from build123d import *

# Parameters (mm, degrees)
SKETCH1_R           = 24.15
SKETCH1_R_2         = 20.3
BOSS_EXTRUDE1_DEPTH = 70
CUT_EXTRUDE1_START  = -3.2
SKETCH2_R           = 21.65
SKETCH2_R_2         = 20.3
CUT_EXTRUDE1_DEPTH  = 3.2
SKETCH3_R           = 60
SKETCH3_R_2         = 8.4
BOSS_EXTRUDE2_DEPTH = 10


with BuildPart() as part:
    # Sketch1 → Boss-Extrude1 (new body)
    with BuildSketch(Plane.XY):
        Circle(SKETCH1_R)
        Circle(SKETCH1_R_2, mode=Mode.SUBTRACT)
    extrude(amount=BOSS_EXTRUDE1_DEPTH)

    # Sketch2 → Cut-Extrude1 (cut)
    with BuildSketch(Plane.XY.offset(70).offset(CUT_EXTRUDE1_START)):
        Circle(SKETCH2_R)
        Circle(SKETCH2_R_2, mode=Mode.SUBTRACT)
    extrude(amount=CUT_EXTRUDE1_DEPTH, mode=Mode.SUBTRACT)

    # Sketch3 → Boss-Extrude2 (add)
    with BuildSketch(Plane.XY.offset(70)):
        Circle(SKETCH3_R)
        Circle(SKETCH3_R_2, mode=Mode.SUBTRACT)
    extrude(amount=BOSS_EXTRUDE2_DEPTH)


solid = part.part
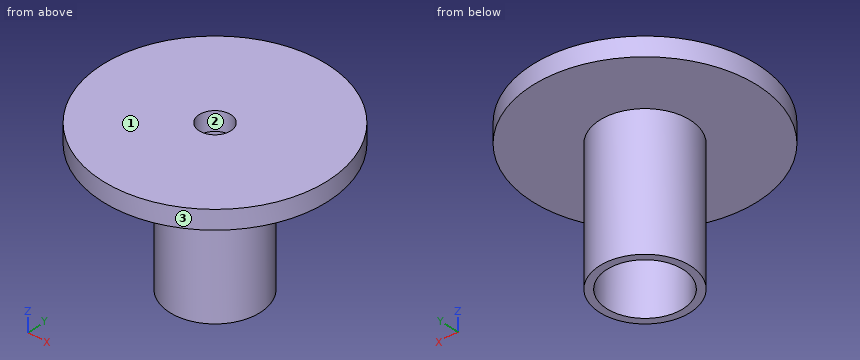
CAD build for the part. Positions are in the model's coordinates, mm. Face numbers are marked on the shaded views. Round coordinates to 2 decimals unless told otherwise and drop trailing zeros. Order: outer loops, then holes, each group sorted by start corner. A loop starts at its lowest first (then second) coordinate and runs counter-clockwise, first axis right, second up. Notation, with made-up numbers: (7, 53.5) -> (13, 53.5) arc R28 ccw to (13, 89.5) -> close; hole circle Ø8 at (-6, 67.25). An arc over 180 degrees is marked (long way). Write each question's results on one line, items separated by ' | '.
1. Cut at C-C (z = 74). Give the cut face in (x, y).
Findings below:
outline: circle Ø120 at (0, 0); hole circle Ø16.8 at (0, 0)
2. Wall check: line 1 along Y through (x, z) = (0, 74); line 2 along Y through (x, z) = (0, 67.7); line 3 along Z through (x, y) = (-8, 19). Give the ranges that are in metal, low to high. Write a range as [from, to].
Findings below:
line 1: y = [-60, -8.4], [8.4, 60] | line 2: y = [-24.15, -21.65], [21.65, 24.15] | line 3: z = [0, 66.8], [70, 80]
3. Pull direction X, two halves, no side cores. Call the marked faces 1, 2 and 3: pulls with the +X half, pulls with the -X half, needs draft (parallel to the pull), parting line crosses it, or undercut.
Findings below:
face 1: needs draft | face 2: undercut | face 3: parting line crosses it
4. Cut at D-D (x = -16.5). Give the cut face in (y, z), plus the area to 3 significant figures.
Findings below:
outline: (-57.69, 70) -> (-17.63, 70) -> (-17.63, 0) -> (-11.83, 0) -> (-11.83, 66.8) -> (-14.02, 66.8) -> (-14.02, 70) -> (14.02, 70) -> (14.02, 66.8) -> (11.83, 66.8) -> (11.83, 0) -> (17.63, 0) -> (17.63, 70) -> (57.69, 70) -> (57.69, 80) -> (-57.69, 80) -> close | area: 1,950 mm²
5. Flat gauge pins, fed straight in: P1, Ø10, axis at x = -13, z = 53.5, coming from the +Y side; P2, Ø2, axis at x = 39.5, y = -36.5, coming from the -Z side; P3, Ø8, axis at y = -37, z = 68.5, coming from the -X side. Where does each tip first touch, or does it go through?
Findings below:
P1: stops at y = 22.79 | P2: stops at z = 70 | P3: stops at x = -49.92
6. Cut at A-A (x = 0). Give the cut face in (y, z).
Findings below:
outline: (-60, 70) -> (-24.15, 70) -> (-24.15, 0) -> (-20.3, 0) -> (-20.3, 66.8) -> (-21.65, 66.8) -> (-21.65, 70) -> (-8.4, 70) -> (-8.4, 80) -> (-60, 80) -> close; (8.4, 70) -> (21.65, 70) -> (21.65, 66.8) -> (20.3, 66.8) -> (20.3, 0) -> (24.15, 0) -> (24.15, 70) -> (60, 70) -> (60, 80) -> (8.4, 80) -> close
